Could you check a few things on this model? Use its own coordinates, in mm. Face numbers are marked on the shaded views. Coordinates: 2 decimals unless noted, no trailing zeros. Order: outer loops, then holes, each group sorted by start corner. A loop starts at its lowest first (then second) coordinate and runs counter-clockwise, first axis right, second up. Notation, with made-up numbers: (59.5, 70.25) - (77.5, 70.25) arc R15 ccw to (77.5, 76.25) - close; hole circle Ø7 at (-14, 14.25). An arc over 180 degrees is marked (long way). Answer as a JSON object with one key per item and string values. Group by question number.
(1) Imagine slicing it at A-A, the plane x = -15. Write out the boundary of the cut face in (y, z) (3 decimals).
(2) Imagine slicing it at C-C, the plane z = 19.5. Write out the boundary of the cut face in (x, y) (3 decimals).
(3) Please list where these lines run through material, in increasing order: probe 1 along X at (y, z) = (-23.25, 15) (3 decimals); probe 2 along Z at (x, y) = (-15, -21.5) (3 decimals).
(4) Imagine slicing it at B-B, the plane y = -15.5. Write out the boundary of the cut face in (x, z) (3 decimals).
(5) We'd pull the mould along Y, two halves only. Please class the marked faces 1, 2 and 3: pulls with the +Y half, pulls with the -Y half, needs draft (parallel to the pull), parting line crosses it, or undercut.
(6) Imagine slicing it at D-D, the plane y = -8.5. Write out the boundary of the cut face in (x, z) (3 decimals), and give its area (3 significant figures).
(7) Will these pins go through, and if not, where does the flat tip stop? P1, Ø3, axis at x = -12, y = -16, coming from the -Z side; P2, Ø4, axis at x = -15, y = -15, coming from the +Z side.
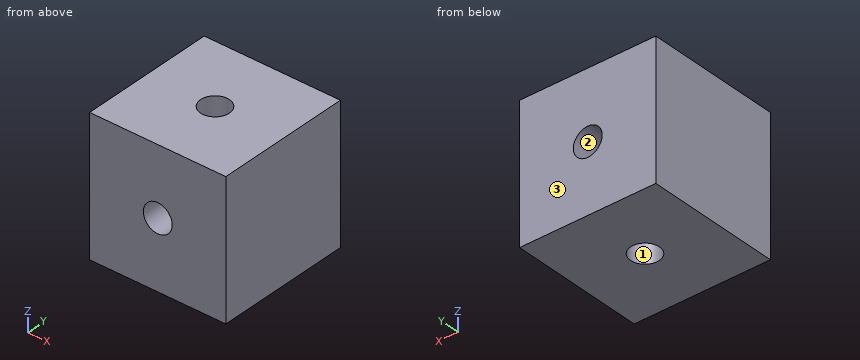
from build123d import *

# Parameters (mm, degrees)
F0_W     = 30
F0_H     = 30
F1_DEPTH = 30
F2_R     = 3.175
F3_DEPTH = 30.001
F4_R     = 3.175
F5_DEPTH = 30.001


with BuildPart() as f1:
    # F0 (on Front) → F1 (new body)
    with BuildSketch(Plane.XZ):
        with Locations((-15, 15)):
            Rectangle(F0_W, F0_H)
    extrude(amount=F1_DEPTH)

    # F2 (on face) → F3 (cut, through all)
    with BuildSketch(Plane(origin=(0, 0, 0), x_dir=(-1, 0, 0), z_dir=(0, 1, 0))):
        with Locations((15, 15)):
            Circle(F2_R)
    extrude(amount=-F3_DEPTH, mode=Mode.SUBTRACT)

    # F4 (on face) → F5 (cut, through all)
    with BuildSketch(Plane(origin=(0, 0, 0), x_dir=(1, 0, 0), z_dir=(0, 0, -1))):
        with Locations((-15, 15)):
            Circle(F4_R)
    extrude(amount=-F5_DEPTH, mode=Mode.SUBTRACT)


solid = f1.part
Result set:
{
 "1": {"outline": "(-30, 0) - (-18.175, 0) - (-18.175, 11.825) - (-30, 11.825) - close; (-30, 18.175) - (-18.175, 18.175) - (-18.175, 30) - (-30, 30) - close; (-11.825, 0) - (0, 0) - (0, 11.825) - (-11.825, 11.825) - close; (-11.825, 18.175) - (0, 18.175) - (0, 30) - (-11.825, 30) - close"},
 "2": {"outline": "(-30, -30) - (0, -30) - (0, 0) - (-30, 0) - close; hole circle Ø6.35 at (-15, -15)"},
 "3": {"probe 1": "x = -30 to -18.175, -11.825 to 0", "probe 2": "z = 0 to 11.825, 18.175 to 30"},
 "4": {"outline": "(-30, 0) - (-18.135, 0) - (-18.135, 14.5) arc R3.175 cw to (-18.135, 15.5) - (-18.135, 30) - (-30, 30) - close; (-11.865, 0) - (0, 0) - (0, 30) - (-11.865, 30) - (-11.865, 15.5) arc R3.175 cw to (-11.865, 14.5) - close"},
 "5": {"face 1": "undercut", "face 2": "needs draft", "face 3": "pulls with the +Y half"},
 "6": {"outline": "(-30, 0) - (0, 0) - (0, 30) - (-30, 30) - close; hole circle Ø6.35 at (-15, 15)", "area": "868 mm^2"},
 "7": {"P1": "stops at z = 0", "P2": "passes through"}
}
